```python
from build123d import *

# Parameters (mm, degrees)
F0_R     = 8.25
F0_R_2   = 1.75
F1_DEPTH = 3
F2_R     = 2
F3_R     = 5


# Not quite as in the source:
# - a feature names something its author has since deleted; it is built from what else it names


with BuildPart() as f1:
    # F0 (on Top) → F1 (new body)
    with BuildSketch(Plane.XY):
        with BuildLine():
            Line((-10.5, -2.6809513237), (-10.5, 0))
            Line((-10.5, 0), (-10.5, 2.6809513237))
            ThreePointArc((-10.5, 2.6809513237), (-11.4360102659, 3.243983813), (-12.5, 3.4910600109))
            Line((-12.5, 3.4910600109), (-12.5, 1.7320508076))
            ThreePointArc((-12.5, 1.7320508076), (-11.4271243445, 1.1456439237), (-11, 0))
            ThreePointArc((-11, 0), (-11.4271243445, -1.1456439237), (-12.5, -1.7320508076))
            Line((-12.5, -1.7320508076), (-12.5, -3.4910600109))
            ThreePointArc((-12.5, -3.4910600109), (-11.4360102659, -3.243983813), (-10.5, -2.6809513237))
        make_face()
        with BuildLine():
            Line((-12.5, 1.7320508076), (-12.5, 3.4910600109))
            ThreePointArc((-12.5, 3.4910600109), (-16.25, 0), (-12.5, -3.4910600109))
            Line((-12.5, -3.4910600109), (-12.5, -1.7320508076))
            ThreePointArc((-12.5, -1.7320508076), (-14.5, 0), (-12.5, 1.7320508076))
        make_face()
        with BuildLine():
            Line((-10.5, 2.6809513237), (-10.5, 5.5))
            Line((-10.5, 5.5), (-12.5, 5.5))
            Line((-12.5, 5.5), (-12.5, 3.4910600109))
            ThreePointArc((-12.5, 3.4910600109), (-11.4360102659, 3.243983813), (-10.5, 2.6809513237))
        make_face()
        with BuildLine():
            ThreePointArc((-10.2181372549, 2.4165411314), (-9.3247712996, 4.8268665001), (-7.8725304742, 6.9478963675))
            Line((-7.8725304742, 6.9478963675), (-10.5, 5.5))
            Line((-10.5, 5.5), (-10.5, 2.6809513237))
            ThreePointArc((-10.5, 2.6809513237), (-10.3554163168, 2.5526396111), (-10.2181372549, 2.4165411314))
        make_face()
        with BuildLine():
            Line((-7.2260237528, 5.7746931281), (-7.8725304742, 6.9478963675))
            ThreePointArc((-7.8725304742, 6.9478963675), (-9.3247712996, 4.8268665001), (-10.2181372549, 2.4165411314))
            ThreePointArc((-10.2181372549, 2.4165411314), (-9.5010371187, 1.301629823), (-9.25, 0))
            ThreePointArc((-9.25, 0), (-8.729353347, 3.0595571809), (-7.2260237528, 5.7746931281))
        make_face()
        with BuildLine():
            ThreePointArc((6.6767394005, 6.401847466), (6.5063300085, 7.2895956499), (6.5689658587, 8.1913788551))
            ThreePointArc((6.5689658587, 8.1913788551), (-0.9007676454, 10.4612913949), (-7.8725304742, 6.9478963675))
            Line((-7.8725304742, 6.9478963675), (-7.2260237528, 5.7746931281))
            ThreePointArc((-7.2260237528, 5.7746931281), (-0.4168440545, 9.2406028502), (6.6767394005, 6.401847466))
        make_face()
        with BuildLine():
            ThreePointArc((9.25, 0), (8.9359851316, 2.3897007611), (8.0152605995, 4.617152534))
            ThreePointArc((8.0152605995, 4.617152534), (7.2, 5.4), (6.6767394005, 6.401847466))
            ThreePointArc((6.6767394005, 6.401847466), (-0.4168440545, 9.2406028502), (-7.2260237528, 5.7746931281))
            ThreePointArc((-7.2260237528, 5.7746931281), (-8.729353347, 3.0595571809), (-9.25, 0))
            ThreePointArc((-9.25, 0), (-8.729353347, -3.0595571809), (-7.2260237528, -5.7746931281))
            ThreePointArc((-7.2260237528, -5.7746931281), (-0.4168440545, -9.2406028502), (6.6767394005, -6.401847466))
            ThreePointArc((6.6767394005, -6.401847466), (7.2, -5.4), (8.0152605995, -4.617152534))
            ThreePointArc((8.0152605995, -4.617152534), (8.9359851316, -2.3897007611), (9.25, 0))
        make_face()
        Circle(F0_R, mode=Mode.SUBTRACT)
        with BuildLine():
            Line((-12.5, -5.5), (-10.5, -5.5))
            Line((-10.5, -5.5), (-10.5, -2.6809513237))
            ThreePointArc((-10.5, -2.6809513237), (-11.4360102659, -3.243983813), (-12.5, -3.4910600109))
            Line((-12.5, -3.4910600109), (-12.5, -5.5))
        make_face()
        with BuildLine():
            Line((-10.5, -5.5), (-7.8725304742, -6.9478963675))
            ThreePointArc((-7.8725304742, -6.9478963675), (-9.3247712996, -4.8268665001), (-10.2181372549, -2.4165411314))
            ThreePointArc((-10.2181372549, -2.4165411314), (-10.3554163168, -2.5526396111), (-10.5, -2.6809513237))
            Line((-10.5, -2.6809513237), (-10.5, -5.5))
        make_face()
        with BuildLine():
            ThreePointArc((-10.5, -2.6809513237), (-10.3554163168, -2.5526396111), (-10.2181372549, -2.4165411314))
            ThreePointArc((-10.2181372549, -2.4165411314), (-10.4292962652, -1.2164618415), (-10.5, 0))
            Line((-10.5, 0), (-10.5, -2.6809513237))
        make_face()
        with BuildLine():
            ThreePointArc((-9.25, 0), (-9.5010371187, 1.301629823), (-10.2181372549, 2.4165411314))
            ThreePointArc((-10.2181372549, 2.4165411314), (-10.4292962652, 1.2164618415), (-10.5, 0))
            ThreePointArc((-10.5, 0), (-10.4292962652, -1.2164618415), (-10.2181372549, -2.4165411314))
            ThreePointArc((-10.2181372549, -2.4165411314), (-9.5010371187, -1.301629823), (-9.25, 0))
        make_face()
        with BuildLine():
            ThreePointArc((-10.2181372549, -2.4165411314), (-9.3247712996, -4.8268665001), (-7.8725304742, -6.9478963675))
            Line((-7.8725304742, -6.9478963675), (-7.2260237528, -5.7746931281))
            ThreePointArc((-7.2260237528, -5.7746931281), (-8.729353347, -3.0595571809), (-9.25, 0))
            ThreePointArc((-9.25, 0), (-9.5010371187, -1.301629823), (-10.2181372549, -2.4165411314))
        make_face()
        with BuildLine():
            ThreePointArc((-10.5, 0), (-10.4292962652, 1.2164618415), (-10.2181372549, 2.4165411314))
            ThreePointArc((-10.2181372549, 2.4165411314), (-10.3554163168, 2.5526396111), (-10.5, 2.6809513237))
            Line((-10.5, 2.6809513237), (-10.5, 0))
        make_face()
        with BuildLine():
            ThreePointArc((-7.8725304742, -6.9478963675), (-0.9007676454, -10.4612913949), (6.5689658587, -8.1913788551))
            ThreePointArc((6.5689658587, -8.1913788551), (6.5063300085, -7.2895956499), (6.6767394005, -6.401847466))
            ThreePointArc((6.6767394005, -6.401847466), (-0.4168440545, -9.2406028502), (-7.2260237528, -5.7746931281))
            Line((-7.2260237528, -5.7746931281), (-7.8725304742, -6.9478963675))
        make_face()
        with BuildLine():
            ThreePointArc((6.5689658587, -8.1913788551), (8.4, -6.3), (9.7030341413, -4.0126211449))
            ThreePointArc((9.7030341413, -4.0126211449), (8.8197842263, -4.2049900262), (8.0152605995, -4.617152534))
            ThreePointArc((8.0152605995, -4.617152534), (7.4, -5.55), (6.6767394005, -6.401847466))
            ThreePointArc((6.6767394005, -6.401847466), (6.5063300085, -7.2895956499), (6.5689658587, -8.1913788551))
        make_face()
        with BuildLine():
            ThreePointArc((13.5, -7.5), (12.3675535363, -4.9222703298), (9.7030341413, -4.0126211449))
            ThreePointArc((9.7030341413, -4.0126211449), (8.4, -6.3), (6.5689658587, -8.1913788551))
            ThreePointArc((6.5689658587, -8.1913788551), (10.3474050269, -10.982715858), (13.5, -7.5))
        make_face()
        with Locations((10, -7.5)):
            Circle(F0_R_2, mode=Mode.SUBTRACT)
        with BuildLine():
            ThreePointArc((6.6767394005, -6.401847466), (7.4, -5.55), (8.0152605995, -4.617152534))
            ThreePointArc((8.0152605995, -4.617152534), (7.2, -5.4), (6.6767394005, -6.401847466))
        make_face()
        with BuildLine():
            ThreePointArc((9.7030341413, -4.0126211449), (10.2988314503, -2.0455001242), (10.5, 0))
            ThreePointArc((10.5, 0), (10.2988314503, 2.0455001242), (9.7030341413, 4.0126211449))
            ThreePointArc((9.7030341413, 4.0126211449), (8.8197842263, 4.2049900262), (8.0152605995, 4.617152534))
            ThreePointArc((8.0152605995, 4.617152534), (8.9359851316, 2.3897007611), (9.25, 0))
            ThreePointArc((9.25, 0), (8.9359851316, -2.3897007611), (8.0152605995, -4.617152534))
            ThreePointArc((8.0152605995, -4.617152534), (8.8197842263, -4.2049900262), (9.7030341413, -4.0126211449))
        make_face()
        with BuildLine():
            ThreePointArc((6.6767394005, 6.401847466), (7.2, 5.4), (8.0152605995, 4.617152534))
            ThreePointArc((8.0152605995, 4.617152534), (7.4, 5.55), (6.6767394005, 6.401847466))
        make_face()
        with BuildLine():
            ThreePointArc((8.0152605995, 4.617152534), (8.8197842263, 4.2049900262), (9.7030341413, 4.0126211449))
            ThreePointArc((9.7030341413, 4.0126211449), (8.4, 6.3), (6.5689658587, 8.1913788551))
            ThreePointArc((6.5689658587, 8.1913788551), (6.5063300085, 7.2895956499), (6.6767394005, 6.401847466))
            ThreePointArc((6.6767394005, 6.401847466), (7.4, 5.55), (8.0152605995, 4.617152534))
        make_face()
        with BuildLine():
            ThreePointArc((6.5689658587, 8.1913788551), (8.4, 6.3), (9.7030341413, 4.0126211449))
            ThreePointArc((9.7030341413, 4.0126211449), (12.3675535363, 4.9222703298), (13.5, 7.5))
            ThreePointArc((13.5, 7.5), (10.3474050269, 10.982715858), (6.5689658587, 8.1913788551))
        make_face()
        with Locations((10, 7.5)):
            Circle(F0_R_2, mode=Mode.SUBTRACT)
    extrude(amount=F1_DEPTH)

    # F2
    f2_edges = [f1.edges().sort_by_distance(p)[0] for p in [
        (-12.5, -3.49106, 1.5),
        (-12.5, 3.49106, 1.5),
    ]]
    fillet(f2_edges, radius=F2_R)

    # F3
    f3_edges = [f1.edges().sort_by_distance(p)[0] for p in [
        (6.568966, -8.191379, 1.5),
        (9.703034, -4.012621, 1.5),
        (9.703034, 4.012621, 1.5),
        (6.568966, 8.191379, 1.5),
    ]]
    fillet(f3_edges, radius=F3_R)


solid = f1.part
```
Could you check a few things on this model? Use its own coordinates, in mm. A direction names the side the tool comes from. Round coordinates to 2 decimals unless told otherwise and drop trailing zeros. Loops run counter-clockwise (first coordinate to the right, second up) from the corner with the lowest first, then second, coordinate; pieces in that order, holes last. Notation, with made-up numbers: (87, -7) - (128, -7) arc R17 cw to (128, 26) - close; hole circle Ø11 at (35.25, 89.25). An arc over 180 degrees is marked (long way). Answer in a Markdown table with one row per item. Add a question column.
(1) If we section it at A-A (x = 0): Please give me the cut outline in (y, z), plus the area to 3 significant figures.
(2) I'm going to push flat-ended pins straight in: pin 1 (1 mm diameter, centred on x = -11.5, z = 2, fed in from -Y); pin 2 (1 mm diameter, centred on x = -6.5, z = 1.5, fed in from -Y); pin 3 (1 mm diameter, centred on x = -12, z = 1.5, fed in from +Y). Where does each tip first touch, or does it pass through?
(3) If we mould it in two halves opening along X, with no side actions, what happens to faces 1 (the face through (-8, 3, 0)), 2 (the face through (-9.205, -6.214, 1.479)), 3 (the face through (10.81, -9.05, 1.48))? For each: pulls with the +X half, pulls with the -X half, needs draft (parallel to the pull), parting line crosses it, or undercut.
(4) I need wall thicknesses on line 1 along Y through (x, z) = (10, 1.4); line 2 along Y through (x, z) = (11.25, 1.65); line 3 along X through (y, z) = (1, 0.45). Which ranges of each line are inside material? Lowest first, please.
(5) For faces 4 (the face through (-11, 5.5, 1)), 5 (the face through (-16.25, 0.06, 1.48)), 6 (the face through (-12, -5.5, 1)), which set-ups out of +Z, -Z, +X, -X, +Y, -Y let a thin tool reach every point of the face, with its end or its side?
(6) If we section it at C-C (z = 2.1): State how many separate pieces and enclosed holes the cut face has, plus the area to 3 significant figures.
(7) If we section it at B-B (x = 3.25): Please give me the cut outline in (y, z), plus the area to 3 significant figures.
Model answer:
| question | item | result |
|---|---|---|
| 1 | outline | (-10.5, 0) - (-8.25, 0) - (-8.25, 3) - (-10.5, 3) - close; (8.25, 0) - (10.5, 0) - (10.5, 3) - (8.25, 3) - close |
| 1 | area | 13.5 mm² |
| 2 | pin 1 | stops at y = -5.5 |
| 2 | pin 2 | stops at y = -8.62 |
| 2 | pin 3 | stops at y = 5.5 |
| 3 | face 1 | needs draft |
| 3 | face 2 | pulls with the -X half |
| 3 | face 3 | undercut |
| 4 | line 1 | y = -11 to -9.25, -5.75 to 5.75, 9.25 to 11 |
| 4 | line 2 | y = -10.77 to -8.72, -6.28 to -3.68, 3.68 to 6.28, 8.72 to 10.77 |
| 4 | line 3 | x = -16.1 to -14.19, -11.31 to -8.19, 8.19 to 10.47 |
| 5 | face 4 | +Z, -Z, -X, +Y |
| 5 | face 5 | +Z, -Z, -X |
| 5 | face 6 | +Z, -Z, -X, -Y |
| 6 | separate pieces | 1 |
| 6 | enclosed holes | 4 |
| 6 | area | 230 mm² |
| 7 | outline | (-9.98, 0) - (-7.58, 0) - (-7.58, 3) - (-9.98, 3) - close; (7.58, 0) - (9.98, 0) - (9.98, 3) - (7.58, 3) - close |
| 7 | area | 14.4 mm² |
